Here's how the part is built. I have some questions about the finished solid (model axes, mm). Give positions to 0.01 mm unless a question says otherwise; leave off trailing zeros. Write each loop counter-clockwise with the first axis right and the second up, starting at its lowest first coordinate (ties: lowest second). Pieces come first, ordered by that corner, then holes. Notation, with made-up numbers: (31, 82) -> (58, 82) arc R24 ccw to (58, 121) -> close; hole circle Ø6 at (50.5, 27). An arc over 180 degrees is marked (long way). Put each result on its own line as item: value. Start each with the question number.
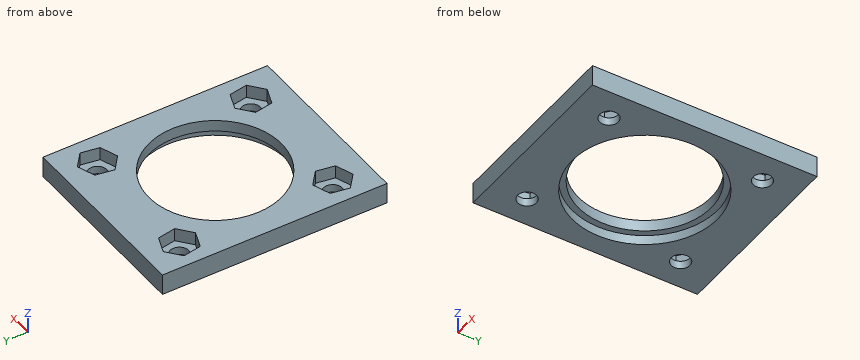
from build123d import *

# Parameters (mm, degrees)
SKETCH2_R           = 11.625
BOSS_EXTRUDE1_DEPTH = 2
SKETCH3_R           = 12.725
BOSS_EXTRUDE2_DEPTH = 1.7
CUT_EXTRUDE1_DEPTH  = 2.3
SKETCH5_R           = 1.65
CUT_EXTRUDE2_DEPTH  = 1.4


with BuildPart() as part:
    # Sketch2 → Boss-Extrude1 (new body)
    with BuildSketch(Plane.XY):
        Polygon((-16.247566177, -19.702007889), (-16.252434142, 19.697992436), (16.34566541, 19.70202001), (16.350533375, -19.697980315), align=None)
        Circle(SKETCH2_R, mode=Mode.SUBTRACT)
    extrude(amount=-BOSS_EXTRUDE1_DEPTH)

    # Sketch3 → Boss-Extrude2 (add)
    with BuildSketch(Plane(origin=(0, 0, -2), x_dir=(-1, 0, 0), z_dir=(0, 0, -1))):
        Polygon((-16.350533375, -19.697980315), (16.247566177, -19.702007889), (16.252434142, 19.697992436), (-16.34566541, 19.70202001), align=None)
        Circle(SKETCH3_R, mode=Mode.SUBTRACT)
    extrude(amount=BOSS_EXTRUDE2_DEPTH)

    # Sketch4 → Cut-Extrude1 (cut)
    with BuildSketch(Plane.XY):
        Polygon((10.632742825, -10.278526808), (8.144960808, -12.343538665), (8.689422526, -15.530527019), (11.721666262, -16.652503517), (14.209448279, -14.58749166), (13.664986561, -11.400503306), align=None)
        Polygon((13.664986561, 11.400503306), (10.632742825, 10.278526808), (8.144960808, 12.343538665), (8.689422526, 15.530527019), (11.721666262, 16.652503517), (14.209448279, 14.58749166), align=None)
        Polygon((-13.664986561, 11.400503306), (-10.632742825, 10.278526808), (-8.144960808, 12.343538665), (-8.689422526, 15.530527019), (-11.721666262, 16.652503517), (-14.209448279, 14.58749166), align=None)
        Polygon((-13.664986561, -11.400503306), (-10.632742825, -10.278526808), (-8.144960808, -12.343538665), (-8.689422526, -15.530527019), (-11.721666262, -16.652503517), (-14.209448279, -14.58749166), align=None)
    extrude(amount=-CUT_EXTRUDE1_DEPTH, mode=Mode.SUBTRACT)

    # Sketch5 → Cut-Extrude2 (cut)
    with BuildSketch(Plane(origin=(0, 0, -3.7), x_dir=(-1, 0, 0), z_dir=(0, 0, -1))):
        with Locations((-11.177204543, -13.465515163)):
            Circle(SKETCH5_R)
        with Locations((-11.177204543, 13.465515163)):
            Circle(SKETCH5_R)
        with Locations((11.177204543, 13.465515163)):
            Circle(SKETCH5_R)
        with Locations((11.177204543, -13.465515163)):
            Circle(SKETCH5_R)
    extrude(amount=-CUT_EXTRUDE2_DEPTH, mode=Mode.SUBTRACT)


solid = part.part
1) I want a section at A-A, the plane z = -1.5. State how many separate pieces and enclosed holes the cut face has, and give its area (3 significant figures).
2) I want a section at B-B, the plane x = 0. Write out the boundary of the cut face in (y, z) (3 decimals).
3) I need wall thicknesses on probe 1 along X at (y, z) = (-13, -3.3); probe 2 along Y at (x, z) = (0, -2.8) (3 decimals); probe 3 along X at (y, z) = (12, -0.5). Which ranges of each line are inside material? Lowest first, please.
4) I'm going to push flat-ended pins straight in: pin 1 Ø2 at (y, z) = (-9, -1.5) entering from -X; pin 2 Ø1.5 at (x, y) = (10, -13) entering from +Z. Where does each tip first touch, or does it pass through?
5) I want a section at C-C, the plane y = -9.5. Write out the boundary of the cut face in (x, z), and give its area (3 significant figures).
Established:
1. separate pieces: 1
1. enclosed holes: 5
1. area: 751 mm2
2. outline: (-19.7, -3.7) -> (-12.725, -3.7) -> (-12.725, -2) -> (-11.625, -2) -> (-11.625, 0) -> (-19.7, 0) -> close; (11.625, -2) -> (12.725, -2) -> (12.725, -3.7) -> (19.7, -3.7) -> (19.7, 0) -> (11.625, 0) -> close
3. probe 1: x = -16.25 to -12.76, -9.59 to 9.59, 12.76 to 16.35
3. probe 2: y = -19.7 to -12.725, 12.725 to 19.7
3. probe 3: x = -16.25 to -13.77, -8.56 to 8.56, 13.77 to 16.35
4. pin 1: stops at x = -16.25
4. pin 2: stops at z = -2.3
5. outline: (-16.25, -3.7) -> (-8.47, -3.7) -> (-8.47, -2) -> (-6.7, -2) -> (-6.7, 0) -> (-16.25, 0) -> close; (6.7, -2) -> (8.47, -2) -> (8.47, -3.7) -> (16.35, -3.7) -> (16.35, 0) -> (6.7, 0) -> close
5. area: 65.0 mm2
